```python
from build123d import *

# Parameters (mm, degrees)
SKETCH_1_W      = 10
SKETCH_1_H      = 3
EXTRUDE_1_DEPTH = 170


with BuildPart() as part:
    # 草图1 → 凸台-拉伸1 (new body)
    with BuildSketch(Plane(origin=(0, 0, 0), x_dir=(1, 0, 0), z_dir=(0, 1, 0))):
        Polygon((-69.608677765, -77.709177727), (-70.851318452, -77.709177727), (-70.851318452, -74.709177727), (14.001495291, 10.143636016), (16.122815634, 8.022315672), align=None)
        with Locations((-75.851318452, -76.209177727)):
            Rectangle(SKETCH_1_W, SKETCH_1_H)
    extrude(amount=EXTRUDE_1_DEPTH)


solid = part.part
```
The listing builds one solid part. Answer for the finished solid, in the listing's coordinates (mm). A direction names the side the tool comes from. Coordinates: 2 decimals unless noted, no trailing zeros. Loops run counter-clockwise (first coordinate to the right, second up) from the corner with the lowest first, then second, coordinate; pieces in that order, holes last. Notation, with made-up numbers: (29.5, -20.5) - (39.5, -20.5) arc R20 ccw to (39.5, 5.5) - close; hole circle Ø5 at (54.5, -25). An arc over 180 degrees is marked (long way). Use a Markdown table: item, result. Add a question column.
1) The part is cut by section A-A, the plane y = 70. Give the vertices of the cut face in (x, z).
2) Given pin 1 (12 mm diameter, centred on y = 87.5, z = 51, fed in from +X); pin 2 (2 mm diameter, centred on y = 33, z = 0.5, fed in from +X); pin 3 (2 mm diameter, centred on x = -7, y = 148, fed in from -Z), each flat-ended and moving along its own axis, determine where each tip first touches the part or whether it passes through.
3) Find the intervals of material crossed by line 1 (Z direction, x = -21.5, y = 149); line 2 (Z direction, x = -6.5, y = 49), in increasing order.
4) The part is cut by section C-C, the plane z = 12.5. Give the vertices of the cut face in (x, y).
5) The part is cut by section B-B, the plane x = -75. Give the vertices of the cut face in (y, z), and give its area (3 significant figures).
6) For faces 1 (the flat face through (-76, 84, 74.709)), 2 (the flat face through (-75, 84, 77.709)), determine the directions among +Z, -Z, +X, -X, +Y, -Y from which every point of the face is accessible in a straight line to the end or side of a thin tool.
Here are the results:
| question | item | result |
|---|---|---|
| 1 | outline | (-80.85, 74.71) - (-70.85, 74.71) - (14, -10.14) - (16.12, -8.02) - (-69.61, 77.71) - (-80.85, 77.71) - close |
| 2 | pin 1 | stops at x = -36.9 |
| 2 | pin 2 | stops at x = 8.6 |
| 2 | pin 3 | stops at z = 9.86 |
| 3 | line 1 | z = 25.36 to 29.6 |
| 3 | line 2 | z = 10.36 to 14.6 |
| 4 | outline | (-8.64, 0) - (-4.4, 0) - (-4.4, 170) - (-8.64, 170) - close |
| 5 | outline | (0, 74.71) - (170, 74.71) - (170, 77.71) - (0, 77.71) - close |
| 5 | area | 510 mm^2 |
| 6 | face 1 | -Z, -X, +Y, -Y |
| 6 | face 2 | +Z, +X, -X, +Y, -Y |
